For this review, take the finished solid that the model builds, in its own axes (mm). A direction names the side the tool comes from. Give positions to 0.01 mm unless a question says otherwise; leave off trailing zeros. Write each loop counter-clockwise with the first axis right and the second up, starting at its lowest first coordinate (ties: lowest second). Pieces come first, ordered by that corner, then holes. Notation, with made-up numbers: (5.25, 82.5) -> (40.25, 82.5) arc R22 cw to (40.25, 95.5) -> close; hole circle Ø9 at (-7.75, 16). An arc over 180 degrees is marked (long way). Answer as CSV lines item,"result".
Autodesk Inventor part; units mm, degrees
ref_plane "YZ Plane" through (0, 0, 0) normal (1, 0, 0) x (0, 1, 0)
ref_plane "XZ Plane" through (0, 0, 0) normal (0, 1, 0) x (-1, 0, 0)
ref_plane "XY Plane" through (0, 0, 0) normal (0, 0, 1) x (1, 0, 0)
sketch "Sketch1" plane through (0, 0, 0) normal (0, 0, 1) x (1, 0, 0)
  line L0 (-30, -30) -> (30, -30)
  line L1 (30, -30) -> (30, 30)
  line L2 (30, 30) -> (-30, 30)
  line L3 (-30, 30) -> (-30, -30)
  line L4 (-30, -30) -> (30, 30) construction
  line L5 (30, -30) -> (-30, 30) construction
  line L6 (30, 30) -> (25, 30) construction
  line L7 (25, 30) -> (25, 25) construction
  line L8 (-30, 30) -> (-25, 30) construction
  line L9 (-25, 30) -> (-25, 25) construction
  line L10 (-30, -30) -> (-30, -25) construction
  line L11 (-30, -25) -> (-25, -25) construction
  line L12 (30, -30) -> (30, -25) construction
  line L13 (30, -25) -> (25, -25) construction
  circle A0 centre (-25, 25) radius 1.5
  circle A1 centre (25, 25) radius 1.5
  circle A2 centre (25, -25) radius 1.5
  circle A3 centre (-25, -25) radius 1.5
  point P0 (0, 0)
  dimension "d0" = 60
  dimension "d1" = 60
  dimension "d2" = 5
  dimension "d3" = 5
  dimension "d4" = 5
  dimension "d5" = 5
  dimension "d6" = 5
  dimension "d7" = 5
  dimension "d8" = 5
  dimension "d9" = 5
  dimension "d10" = 3
  dimension "d11" = 3
  dimension "d12" = 3
  dimension "d13" = 3
extrude "Block" add sketch "Sketch1" along normal blind 60
sketch "Sketch2" plane through (30, -30, 0) normal (1, 0, 0) x (0, 0, -1)
  line L0 (0, 60) -> (-60, 60)
  line L1 (-30, 60) -> (-15.25, 60)
  line L2 (-30, 60) -> (-44.75, 60)
  line L3 (-30, 60) -> (-30, 51.1) construction
  line L4 (-30, 51.1) -> (-8.25, 51.1)
  line L5 (-30, 51.1) -> (-51.75, 51.1)
  line L6 (-51.75, 51.1) -> (-51.75, 53.1)
  line L7 (-8.25, 51.1) -> (-8.25, 53.1)
  line L8 (-8.25, 53.1) -> (-15.25, 60)
  line L9 (-51.75, 53.1) -> (-44.75, 60)
  point P0 (0, 30)
  dimension "d17" = 14.75
  dimension "d18" = 14.75
  dimension "d19" = 8.9
  dimension "d20" = 21.75
  dimension "d21" = 21.75
  dimension "d22" = 2
  dimension "d23" = 2
extrude "Tripod Slot" cut sketch "Sketch2" against normal blind 60
sketch "Sketch3" plane through (0, 0, 60) normal (0, 0, 1) x (1, 0, 0)
  circle A0 centre (-25, -25) radius 1.5 construction
  line L0 (-25, -25) -> (-25, -20) construction
  line L1 (-25, -25) -> (-20, -25) construction
  line L2 (25.1388, -25) -> (25.1388, -20) construction
  line L3 (25.1388, -25) -> (30.1388, -25) construction
  line L4 (-25, 24.9661) -> (-25, 17.4661) construction
  line L5 (-25, 24.9661) -> (-17.5, 24.9661) construction
  line L6 (25.1388, 24.9661) -> (25.1388, 17.4661) construction
  line L7 (25.1388, 24.9661) -> (32.6388, 24.9661) construction
  line L8 (25.1388, 17.4661) -> (30, 17.4661) construction
  line L9 (30, -30) -> (30, 30) construction
  line L10 (-25, 17.4661) -> (-30, 17.4661) construction
  line L11 (-30, 30) -> (-30, -30) construction
  line L12 (-25, -20) -> (-30, -20) construction
  line L13 (25.1388, -20) -> (30, -20) construction
  line L14 (30, 17.4661) -> (5, 17.4661)
  line L15 (30, -20) -> (5, -20)
  line L16 (5, -20) -> (5, 17.4661)
  line L17 (-30, 17.4661) -> (-5, 17.4661)
  line L18 (-30, -20) -> (-5, -20)
  line L19 (-5, -20) -> (-5, 17.4661)
  line L20 (-30, 17.4661) -> (-30, -20)
  line L21 (30, 17.4661) -> (30, -20)
  point P0 (0, 0)
  dimension "d26" = 5
  dimension "d27" = 90
  dimension "d28" = 5
  dimension "d29" = 90
  dimension "d30" = 7.5
  dimension "d31" = 90
  dimension "d32" = 7.5
  dimension "d33" = 90
  dimension "d34" = 25
  dimension "d35" = 25
  dimension "d36" = 25
  dimension "d37" = 25
  dimension "d38" = 90
  dimension "d39" = 90
  dimension "d40" = 4.8612
  dimension "d41" = 4.8612
  dimension "d42" = 55
extrude "Plastic Thinning" cut sketch "Sketch3" against normal blind 60
fillet "Strength" radius 3 10 edges at (30, -20, 30) (5, 17.4661, 30) (-5, 17.4661, 30) (-5, -20, 30) (5, -20, 30) (30, -30, 30) (-30, -30, 30) (-30, -20, 30) (-30, 17.4661, 30) (30, 17.4661, 30)
properties part number "60x60CameraMount"
Q1. To check wall thickness, follow probe 1 along X at (y, z) = (25, 53.25); probe 2 along Y at (x, z) = (-25, 19); probe 3 along Y at (x, z) = (25, 4.25). State the ranges of each line that lie inside material, in increasing order. Write a range as [from, to].
Answer block:
probe 1,"x = [-30, -26.5], [-23.5, 23.5], [26.5, 30]"
probe 2,"y = [-30, -26.5], [-23.5, -20], [17.47, 21.1]"
probe 3,"y = [-30, -26.5], [-23.5, -20], [17.47, 23.5], [26.5, 30]"
Q2. Draft analysis for pull direction Z (two halves, no side actions). For faces 4 (the cylindrical face through (-25.325, 26.464, 55.366)), 5 (the flat face through (0, 7, 0)), 6 (the flat face through (0, 22, 51.75)), state which applies: released by +Z, released by -Z, zero draft, split by the parting line, or undercut.
Answer block:
face 4,"zero draft"
face 5,"released by -Z"
face 6,"undercut"
Q3. Add section A-A (y = -25). Write out the cut boundary in (x, z), plus the area to 3 significant figures.
Answer block:
outline,"(-30, 0) -> (-26.5, 0) -> (-26.5, 60) -> (-30, 60) -> close; (-23.5, 0) -> (23.5, 0) -> (23.5, 60) -> (-23.5, 60) -> close; (26.5, 0) -> (30, 0) -> (30, 60) -> (26.5, 60) -> close"
area,"3,240 mm2"
Q4. Add section B-B (z = 29.5). Write out the cut boundary in (x, y).
Answer block:
outline,"(-30, -27) arc R3 ccw to (-27, -30) -> (27, -30) arc R3 ccw to (30, -27) -> (30, -23) arc R3 ccw to (27, -20) -> (8, -20) arc R3 cw to (5, -17) -> (5, 14.47) arc R3 cw to (8, 17.47) -> (27, 17.47) arc R3 ccw to (30, 20.47) -> (30, 21.1) -> (-30, 21.1) -> (-30, 20.47) arc R3 ccw to (-27, 17.47) -> (-8, 17.47) arc R3 cw to (-5, 14.47) -> (-5, -17) arc R3 cw to (-8, -20) -> (-27, -20) arc R3 ccw to (-30, -23) -> close; hole circle Ø3 at (-25, -25); hole circle Ø3 at (25, -25)"
Q5. Add section C-C (z = 4). Write out the cut boundary in (x, y).
Answer block:
outline,"(-30, -27) arc R3 ccw to (-27, -30) -> (27, -30) arc R3 ccw to (30, -27) -> (30, -23) arc R3 ccw to (27, -20) -> (8, -20) arc R3 cw to (5, -17) -> (5, 14.47) arc R3 cw to (8, 17.47) -> (27, 17.47) arc R3 ccw to (30, 20.47) -> (30, 30) -> (-30, 30) -> (-30, 20.47) arc R3 ccw to (-27, 17.47) -> (-8, 17.47) arc R3 cw to (-5, 14.47) -> (-5, -17) arc R3 cw to (-8, -20) -> (-27, -20) arc R3 ccw to (-30, -23) -> close; hole circle Ø3 at (-25, -25); hole circle Ø3 at (-25, 25); hole circle Ø3 at (25, -25); hole circle Ø3 at (25, 25)"
Q6. Clearance check with flat-ended pins moving along their axes: pin 1 (9.5 mm diameter, centred on y = 3, z = 20, fed in from +X); pin 2 (2 mm diameter, centred on y = 14, z = 42, fed in from -X); pin 3 (5.5 mm diameter, centred on x = 20.5, z = 30, fed in from +Y). State where each tip first meets the part, or that it passes through.
Answer block:
pin 1,"stops at x = 5"
pin 2,"stops at x = -5.05"
pin 3,"stops at y = 21.1"
Q7. Add section D-D (x = -22.5). Write out the cut boundary in (y, z).
Answer block:
outline,"(-30, 0) -> (-20, 0) -> (-20, 60) -> (-30, 60) -> close; (17.47, 0) -> (30, 0) -> (30, 15.25) -> (23.1, 8.25) -> (21.1, 8.25) -> (21.1, 51.75) -> (23.1, 51.75) -> (30, 44.75) -> (30, 60) -> (17.47, 60) -> close"
Q8. For faces 1 (the flat face through (18, 17.466, 30)), 2 (the flat face through (-5, -1, 30)), 3 (the flat face through (0, 21.1, 30)), list the 3-axis set-ups (+Z, -Z, +X, -X, +Y, -Y) from which the entire face can be reached by the end or side of a thin tool; tool diameter is ignored.
Answer block:
face 1,"+Z, -Z, +X"
face 2,"+Z, -Z, -X"
face 3,"+X, -X"
